Work out the finished part from the listing and answer in its coordinate system (mm). A direction names the side the tool comes from. Round coordinates to 2 decimals unless told otherwise and drop trailing zeros. Loops run counter-clockwise (first coordinate to the right, second up) from the corner with the lowest first, then second, coordinate; pieces in that order, holes last.
Autodesk Inventor part; units mm, degrees
ref_plane "YZ Plane" through (0, 0, 0) normal (1, 0, 0) x (0, 1, 0)
ref_plane "XZ Plane" through (0, 0, 0) normal (0, 1, 0) x (-1, 0, 0)
ref_plane "XY Plane" through (0, 0, 0) normal (0, 0, 1) x (1, 0, 0)
sketch "Sketch1" plane through (0, 0, 0) normal (0, 0, 1) x (1, 0, 0)
  line L0 (-177.8, -241.3) -> (177.8, -241.3)
  line L1 (177.8, -241.3) -> (177.8, 241.3)
  line L2 (177.8, 241.3) -> (-177.8, 241.3)
  line L3 (-177.8, 241.3) -> (-177.8, -241.3)
  line L4 (-177.8, -241.3) -> (177.8, 241.3) construction
  line L5 (177.8, -241.3) -> (-177.8, 241.3) construction
  point P0 (0, 0)
  dimension "d0" = 355.6
  dimension "d1" = 482.6
extrude "Extrusion1" add sketch "Sketch1" along normal blind 107.95
sketch "Sketch2" plane through (-177.8, 241.3, 0) normal (0, 1, 0) x (1, 0, 0)
  line L0 (355.6, 0) -> (0, 0)
  line L1 (0, 0) -> (0, -107.95)
  line L2 (355.6, -107.95) -> (0, -107.95)
  line L3 (355.6, 0) -> (355.6, -107.95)
  circle A0 centre (177.8, -53.975) radius 22.225
  line L4 (177.8, -53.975) -> (177.8, -107.95) construction
  line L5 (0, -107.95) -> (355.6, -107.95)
  line L6 (177.8, -53.975) -> (355.6, -53.975) construction
  point P0 (177.8, 0)
  dimension "d4" = 44.45
extrude "Extrusion2" add sketch "Sketch2" along normal blind 590.55 contours A0
sketch "Sketch3" plane through (0, 831.85, 53.975) normal (0, 1, 0) x (1, 0, 0)
  circle A0 centre (0, 0) radius 22.225
  line L0 (-457.2, 53.975) -> (457.2, 53.975)
  line L1 (457.2, 53.975) -> (457.2, -53.975)
  line L2 (457.2, -53.975) -> (-457.2, -53.975)
  line L3 (-457.2, -53.975) -> (-457.2, 53.975)
  circle A1 centre (0, 0) radius 22.225
  line L4 (177.8, 53.975) -> (-177.8, 53.975)
  line L5 (-177.8, 53.975) -> (-177.8, -53.975)
  line L6 (177.8, -53.975) -> (-177.8, -53.975)
  line L7 (177.8, 53.975) -> (177.8, -53.975)
  line L8 (0, 0) -> (0, 53.975) construction
  point P0 (0, 53.975)
  dimension "d7" = 914.4
  dimension "d10" = 107.95
extrude "Extrusion3" add sketch "Sketch3" along normal blind 107.95 contours A0 | L0 L5 L2 L3 | L0 L7 L2 L5 | L0 L1 L2 L7
properties part number "switchbox"
Item 1: Section A-A, the plane x = -34.5 is taken. Give the vertices of the cut face in (y, z).
Item 2: Each of these flat-tipped pins is pushed along its axis until it touches: P1, Ø5, axis at y = 276, z = 76.5, coming from the +X side; P2, Ø10, axis at x = 313, z = 94, coming from the -Y side; P3, Ø2, axis at y = 699, z = 54.5, coming from the -X side (3 decimals). Where does it stop, or does it pass through?
Item 3: Section B-B, the plane y = -50 is taken. Give the vertices of the cut face in (x, z).
Item 4: For faces 4 (the face through (11.948, 532.441, 72.715)), 5 (the face through (-177.8, 3, 53)), 6 (the face through (177.8, -3, 53)), determine the directions among +Z, -Z, +X, -X, +Y, -Y from which every point of the face is accessible in a straight line to the end or side of a thin tool.
Item 5: Section D-D, the plane y = 262.5 is taken. Give the vertices of the cut face in (x, z) (3 decimals).
Item 6: Section C-C, the plane x = -241.5 is taken. Give the vertices of the cut face in (y, z), plus the area to 3 significant figures.
Item 7: Determine the mould class of faces 1 (the face through (-6, 831.85, 77)), 2 (the face through (-2, -241.3, 53)), 3 (the face through (-2, 3, 0)) for opening direction Y: pulls with the +Y half, pulls with the -Y half, needs draft (parallel to the pull), parting line crosses it, or undercut.
Item 8: Straight lines are drawn through the part: line 1 (Y direction, x = -102.5, z = 49); line 2 (Y direction, x = 188, z = 67.5); line 3 (X direction, y = -173, z = 47.5). For each, find the intervals that lie inside material, in ascending order.
Answer below:
1. outline: (-241.3, 0) - (241.3, 0) - (241.3, 107.95) - (-241.3, 107.95) - close; (831.85, 0) - (939.8, 0) - (939.8, 107.95) - (831.85, 107.95) - close
2. P1: stops at x = 9.64
2. P2: stops at y = 831.85
2. P3: stops at x = -22.225
3. outline: (-177.8, 0) - (177.8, 0) - (177.8, 107.95) - (-177.8, 107.95) - close
4. face 4: none
4. face 5: +Z, -Z, -X, -Y
4. face 6: +Z, -Z, +X, -Y
5. outline: circle Ø44.45 at (0, 53.975)
6. outline: (831.85, 0) - (939.8, 0) - (939.8, 107.95) - (831.85, 107.95) - close
6. area: 11,700 mm2
7. face 1: undercut
7. face 2: pulls with the -Y half
7. face 3: needs draft
8. line 1: y = -241.3 to 241.3, 831.85 to 939.8
8. line 2: y = 831.85 to 939.8
8. line 3: x = -177.8 to 177.8
